```python
from build123d import *

# Parameters (mm, degrees)
SKETCH_1_W               = 36
SKETCH_1_H               = 16
EXTRUDE_1_DEPTH          = 7
CUT_EXTRUDE_1_DEPTH      = 26.079872408
CUT_EXTRUDE_1_DEPTH_BACK = 26.079872408
SKETCH_5_R               = 4.9
CUT_EXTRUDE_2_DEPTH      = 0.8
SKETCH_6_R               = 4
CUT_EXTRUDE_3_DEPTH      = 21.505852823
SKETCH_7_W               = 17
SKETCH_7_H               = 2
CUT_EXTRUDE_4_DEPTH      = 0.6
SKETCH_8_W               = 17
SKETCH_8_H               = 2
CUT_EXTRUDE_5_DEPTH      = 0.6
SKETCH_9_R               = 2.9
CUT_EXTRUDE_6_DEPTH      = 21.90454496


with BuildPart() as part:
    # 草图1 → 凸台-拉伸1 (new body)
    with BuildSketch(Plane(origin=(0, 0, 0), x_dir=(1, 0, 0), z_dir=(0, 1, 0))):
        Rectangle(SKETCH_1_W, SKETCH_1_H)
    extrude(amount=EXTRUDE_1_DEPTH)

    # 草图4 → 切除-拉伸1 (cut, two sides: drawn at the far end of the back side and taken through both)
    with BuildSketch(Plane(origin=(0, 0, -8), x_dir=(-1, 0, 0), z_dir=(0, 0, -1)).offset(-CUT_EXTRUDE_1_DEPTH_BACK)):
        Polygon((-8.5, 71.817880295), (-8.5, 7), (-8.5, 6.5), (8.5, 6.5), (8.5, 7), (8.5, 71.817880295), (8.5, 201.453640884), (-8.5, 201.453640884), align=None)
    extrude(amount=CUT_EXTRUDE_1_DEPTH + CUT_EXTRUDE_1_DEPTH_BACK, mode=Mode.SUBTRACT)

    # 草图5 → 切除-拉伸2 (cut)
    with BuildSketch(Plane(origin=(0, 6.5, 0), x_dir=(1, 0, 0), z_dir=(0, 1, 0))):
        with Locations(Location((0, 0, 0), (0, 0, 180))):
            Circle(SKETCH_5_R)
    extrude(amount=-CUT_EXTRUDE_2_DEPTH, mode=Mode.SUBTRACT)

    # 草图6 → 切除-拉伸3 (cut, through all)
    with BuildSketch(Plane(origin=(0, 5.7, 0), x_dir=(1, 0, 0), z_dir=(0, 1, 0))):
        with Locations(Location((0, 0, 0), (0, 0, 180))):
            Circle(SKETCH_6_R)
    extrude(amount=-CUT_EXTRUDE_3_DEPTH, mode=Mode.SUBTRACT)

    # 草图7 → 切除-拉伸4 (cut)
    with BuildSketch(Plane(origin=(0, 6.5, 0), x_dir=(1, 0, 0), z_dir=(0, 1, 0))):
        with Locations((0, 7)):
            Rectangle(SKETCH_7_W, SKETCH_7_H)
    extrude(amount=-CUT_EXTRUDE_4_DEPTH, mode=Mode.SUBTRACT)

    # 草图8 → 切除-拉伸5 (cut)
    with BuildSketch(Plane(origin=(0, 6.5, 0), x_dir=(1, 0, 0), z_dir=(0, 1, 0))):
        with Locations((0, -7)):
            Rectangle(SKETCH_8_W, SKETCH_8_H)
    extrude(amount=-CUT_EXTRUDE_5_DEPTH, mode=Mode.SUBTRACT)

    # 草图9 → 切除-拉伸6 (cut, through all)
    with BuildSketch(Plane(origin=(0, 7, 0), x_dir=(1, 0, 0), z_dir=(0, 1, 0))):
        with Locations(Location((-12, 0, 0), (0, 0, 270))):
            Circle(SKETCH_9_R)
        with Locations(Location((12, 0, 0), (0, 0, 270))):
            Circle(SKETCH_9_R)
    extrude(amount=-CUT_EXTRUDE_6_DEPTH, mode=Mode.SUBTRACT)


solid = part.part
```
Could you check a few things on this model? Use its own coordinates, in mm. A direction names the side the tool comes from. Round coordinates to 2 decimals unless told otherwise and drop trailing zeros. Write each loop counter-clockwise with the first axis right and the second up, starting at its lowest first coordinate (ties: lowest second). Pieces come first, ordered by that corner, then holes.
(1) Suppose I cut it at D-D on z = -2.5. Write out the boundary of the cut face in (x, y).
Findings below:
outline: (-18, 0) - (-13.47, 0) - (-13.47, 7) - (-18, 7) - close; (-10.53, 0) - (-3.12, 0) - (-3.12, 5.7) - (-4.21, 5.7) - (-4.21, 6.5) - (-8.5, 6.5) - (-8.5, 7) - (-10.53, 7) - close; (3.12, 0) - (10.53, 0) - (10.53, 7) - (8.5, 7) - (8.5, 6.5) - (4.21, 6.5) - (4.21, 5.7) - (3.12, 5.7) - close; (13.47, 0) - (18, 0) - (18, 7) - (13.47, 7) - close
(2) Thinking about a two-plate mould opening in Z: for faces 4 (the face through (15.3, 7, -0.1)), 5 (the face through (-13.765, 3.549, -2.301)), 6 (the face through (0, 3, -8)), which applies, +Z half, -Z half, draft (parallel to the pull), parting line (faces both ways), or undercut?
Findings below:
face 4: draft
face 5: undercut
face 6: -Z half
(3) Suppose I cut it at B-B on y = 2.25. Write out the boundary of the cut face in (x, z).
Findings below:
outline: (-18, -8) - (18, -8) - (18, 8) - (-18, 8) - close; hole circle Ø5.8 at (-12, 0); hole circle Ø8 at (0, 0); hole circle Ø5.8 at (12, 0)
(4) Which directions (+Z, -Z, +X, -X, +Y, -Y) give clear straight access to the entire face, cutting with the end or side of a thin tool? Please do faces 1 (the face through (0, 5.9, -7)), 2 (the face through (3.612, 6.106, 3.312)), 3 (the face through (0, 5.9, 7)).
Findings below:
face 1: -Z, +Y
face 2: +Y
face 3: +Z, +Y
(5) Suppose I cut it at C-C on z = -5.5. Write out the boundary of the cut face in (x, y), and give its area (4 significant figures).
Findings below:
outline: (-18, 0) - (18, 0) - (18, 7) - (8.5, 7) - (8.5, 6.5) - (-8.5, 6.5) - (-8.5, 7) - (-18, 7) - close
area: 243.5 mm2
(6) Suppose I cut it at A-A on x = 12. Write out the boundary of the cut face in (y, z), and give its area (3 significant figures).
Findings below:
outline: (0, -8) - (7, -8) - (7, -2.9) - (0, -2.9) - close; (0, 2.9) - (7, 2.9) - (7, 8) - (0, 8) - close
area: 71.4 mm2
(7) For pin 1 (2 mm diameter, centred on x = -3.5, z = -2, fed in from -Y); pin 2 (2 mm diameter, centred on x = -0.5, z = 6.5, fed in from +Y), each with a flat end and sliding along its axis, tell me the tip position at first contact or that it passes through.
Findings below:
pin 1: stops at y = 0
pin 2: stops at y = 6.5
(8) If I drill on probe 1 along X at (y, z) = (6, 2.25); probe 2 along Z at (x, y) = (0, 3.7); probe 3 along Y at (x, z) = (-4, 5.5), over which ranges is the centre line in solid material (lowest first)?
Findings below:
probe 1: x = -18 to -13.83, -10.17 to -4.35, 4.35 to 10.17, 13.83 to 18
probe 2: z = -8 to -4, 4 to 8
probe 3: y = 0 to 6.5
